Answer from the drawing. Dimensions are ordinates in mm from the lowest x, y and z of the part. Coordinates: 2 decimals unless noted, no trailing zeros. Write each loop counter-clockwise with the first axis right and the second up, starting at its lowest first coordinate (ties: lowest second). Pieces come first, ordered by that corner, then holes.
1) Determine the mould class of the marked faces 1, 2 and 3 for opening direction Z: +Z half, -Z half, draft (parallel to the pull), parting line (faces both ways), or undercut.
2) Find the intervals of material crossed by line 1 (X direction, y = 5, z = 11) (1 decimal); line 2 (Z direction, x = 9, y = 7) (1 decimal); line 3 (Z direction, x = 11.5, y = 6.5) (1 decimal), in increasing order.
3) The part is cut by section A-A (z = 11). Determine the outline of the cut face in (x, y) (1 decimal).
4) Each of these flat-tipped pins is pushed along its axis until it touches: pin 1 Ø3 at (x, y) = (6, 2.5) entering from +Z; pin 2 Ø1.9 at (x, z) = (12.5, 11.5) entering from -Y; pin 3 Ø3 at (y, z) = (11.5, 14.5) entering from -X. Where does it stop, or does it pass through?
5) The part is cut by section D-D (y = 10.75). Determine the outline of the cut face in (x, z).
6) The part is cut by section B-B (x = 11). Determine the outline of the cut face in (y, z) (1 decimal), then the cut area to 3 significant figures.
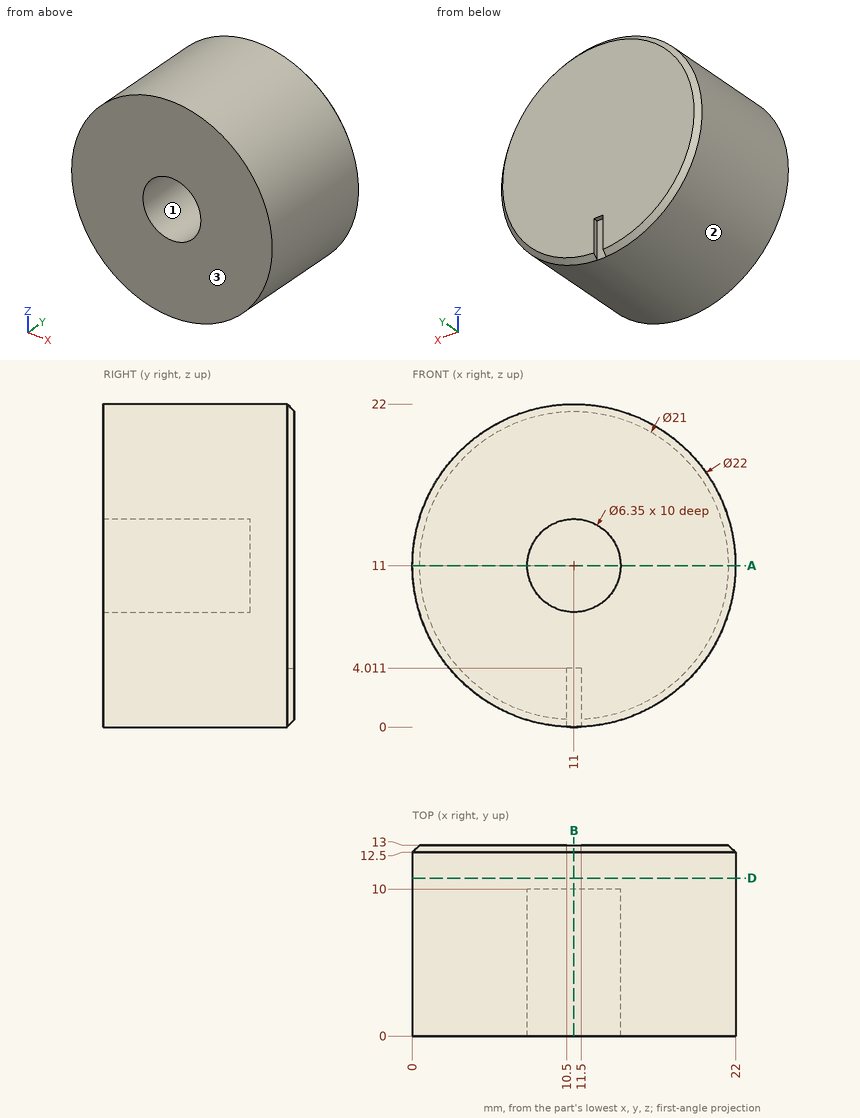
Reported:
1. face 1: undercut
1. face 2: parting line
1. face 3: draft
2. line 1: x = 0 to 7.8, 14.2 to 22
2. line 2: z = 0.2 to 8.5, 13.5 to 21.8
2. line 3: z = 0 to 7.9, 14.1 to 22
3. outline: (0, 0) - (7.8, 0) - (7.8, 10) - (14.2, 10) - (14.2, 0) - (22, 0) - (22, 12.5) - (21.5, 13) - (0.5, 13) - (0, 12.5) - close
4. pin 1: stops at z = 21.43
4. pin 2: stops at y = 10
4. pin 3: stops at x = 0.18
5. outline: circle Ø22 at (11, 11)
6. outline: (0, 0) - (12.5, 0) - (12.5, 4) - (13, 4) - (13, 21.5) - (12.5, 22) - (0, 22) - (0, 14.2) - (10, 14.2) - (10, 7.8) - (0, 7.8) - close
6. area: 220 mm2
